Read the model definition and answer for the solid it produces. Units are mm, in the model's axes. Face numbers are marked on the shaded views. A direction names the side the tool comes from. Give positions to 0.01 mm unless a question says otherwise; leave off trailing zeros. Write each loop counter-clockwise with the first axis right and the second up, starting at its lowest first coordinate (ties: lowest second). Pieces come first, ordered by that corner, then holes. Notation, with made-up numbers: (21, -12) - (41, -12) arc R19 ccw to (41, 11) - close; hole circle Ø8 at (12.25, 8). An arc over 180 degrees is marked (long way). Answer as CSV lines item,"result".
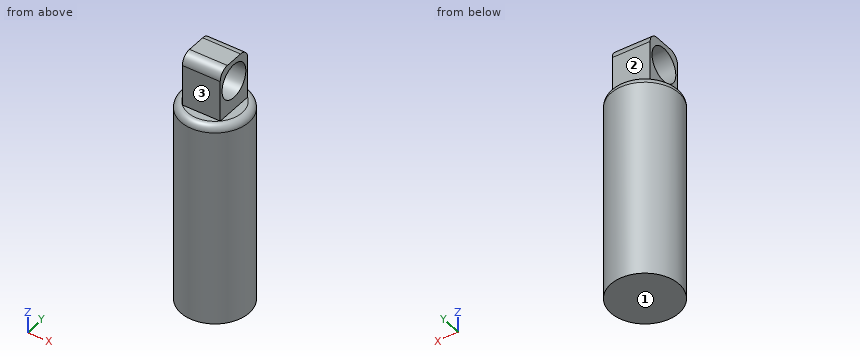
```python
from build123d import *

# Parameters (mm, degrees)
F0_R     = 25.4
F1_DEPTH = 152.4
F2_R     = 5.08
F3_W     = 28.1686
F3_H     = 29.29402
F4_DEPTH = 38.1
F6_R     = 7.62
F5_R     = 12.7
F7_DEPTH = 39.4853


with BuildPart() as f1:
    # F0 (on Top) → F1 (new body)
    with BuildSketch(Plane.XY):
        Circle(F0_R)
    extrude(amount=F1_DEPTH)

    # F2
    f2_edges = [f1.edges().sort_by_distance(p)[0] for p in [
        (-25.4, 0, 152.4),
    ]]
    fillet(f2_edges, radius=F2_R)

    # F3 (on face) → F4 (join)
    with BuildSketch(Plane.XY.offset(152.4)):
        Rectangle(F3_W, F3_H)
    extrude(amount=F4_DEPTH)

    # F6
    f6_edges = [f1.edges().sort_by_distance(p)[0] for p in [
        (0, -14.64701, 190.5),
        (0, 14.64701, 190.5),
    ]]
    fillet(f6_edges, radius=F6_R)

    # F5 (on face) → F7 (cut, through all)
    with BuildSketch(Plane.YZ.offset(14.0843)):
        with Locations((0, 174.101845)):
            Circle(F5_R)
    extrude(amount=-F7_DEPTH, mode=Mode.SUBTRACT)


solid = f1.part
```
(1) For the marked faces 1, 2 and 3, determine the directions among +Z, -Z, +X, -X, +Y, -Y from which every point of the face is accessible in a straight line to the end or side of a thin tool.
Worked out:
face 1,"-Z, +X, -X, +Y, -Y"
face 2,"+Z, +X, -X, +Y"
face 3,"+Z, +X, -X, -Y"
(2) A cutting plane is placed at B-B (x = 0). Write down the section's boundary in (y, z), and give its area (3 significant figures).
Worked out:
outline,"(-25.4, 0) - (25.4, 0) - (25.4, 147.32) arc R5.08 ccw to (20.32, 152.4) - (14.65, 152.4) - (14.65, 182.88) arc R7.62 ccw to (7.03, 190.5) - (-7.03, 190.5) arc R7.62 ccw to (-14.65, 182.88) - (-14.65, 152.4) - (-20.32, 152.4) arc R5.08 ccw to (-25.4, 147.32) - close; hole circle Ø25.4 at (0, 174.1)"
area,"8,320 mm^2"
(3) A cutting plane is placed at A-A (y = 0). Write down the section's boundary in (x, z), and give its area (3 significant figures).
Worked out:
outline,"(-25.4, 0) - (25.4, 0) - (25.4, 147.32) arc R5.08 ccw to (20.32, 152.4) - (14.08, 152.4) - (14.08, 161.4) - (-14.08, 161.4) - (-14.08, 152.4) - (-20.32, 152.4) arc R5.08 ccw to (-25.4, 147.32) - close; (-14.08, 186.8) - (14.08, 186.8) - (14.08, 190.5) - (-14.08, 190.5) - close"
area,"8,090 mm^2"
(4) Each of these flat-tipped pins is pushed along its axis until it touches: P1, Ø22.5, axis at x = 7, z = 167.5, coming from the +Y side; P2, Ø5, axis at y = -7.5, z = 109, coming from the -X side; P3, Ø1.7, axis at x = -4.5, y = 16.5, coming from the +Z side. Where does it stop, or does it pass through?
Worked out:
P1,"stops at y = 14.65"
P2,"stops at x = -24.9"
P3,"stops at z = 152.4"
(5) Find the intervals of material crossed by L1, parallel to Z at x = -3.75, y = 0; L2, parallel to X at y = -6, z = 161.5; L3, parallel to Z at x = -6, y = -6.5, in increasing order.
Worked out:
L1,"z = 0 to 161.4, 186.8 to 190.5"
L2,"x = -14.08 to 14.08"
L3,"z = 0 to 163.19, 185.01 to 190.5"
(6) A cutting plane is placed at C-C (z = 118). Write down the section's boundary in (x, y), and give its area (3 significant figures).
Worked out:
outline,"circle Ø50.8 at (0, 0)"
area,"2,030 mm^2"
